Source: CAD feature listing. Evaluate the final solid. Frame: model axes, mm. A direction names the side the tool comes from. Coordinates: 2 decimals unless noted, no trailing zeros. Order: outer loops, then holes, each group sorted by start corner. A loop starts at its lowest first (then second) coordinate and runs counter-clockwise, first axis right, second up.
```python
from build123d import *

# Parameters (mm, degrees)
SKETCH1_R           = 1.25
SKETCH1_R_2         = 0.5
BOSS_EXTRUDE1_DEPTH = 6
BOSS_EXTRUDE2_DEPTH = 2
CUT_EXTRUDE1_DEPTH  = 1
CUT_EXTRUDE2_DEPTH  = 1
CUT_EXTRUDE3_DEPTH  = 2
CUT_EXTRUDE4_DEPTH  = 1
SKETCH9_R           = 1.5
CUT_EXTRUDE5_DEPTH  = 3


with BuildPart() as part:
    # Sketch1 → Boss-Extrude1 (new body)
    with BuildSketch(Plane.XY):
        with BuildLine():
            Line((2, 0), (14, 0))
            Line((14, 0), (14, 10))
            Line((14, 10), (2, 10))
            ThreePointArc((2, 10), (0.585786438, 9.414213562), (0, 8))
            Line((0, 8), (0, 2))
            ThreePointArc((0, 2), (0.585786438, 0.585786438), (2, 0))
        make_face()
        with Locations((3, 5)):
            Circle(SKETCH1_R, mode=Mode.SUBTRACT)
        with Locations((9, 8)):
            Circle(SKETCH1_R_2, mode=Mode.SUBTRACT)
        with Locations((9, 2)):
            Circle(SKETCH1_R_2, mode=Mode.SUBTRACT)
    extrude(amount=BOSS_EXTRUDE1_DEPTH)

    # Sketch2 → Boss-Extrude2 (add)
    with BuildSketch(Plane(origin=(14, 0, 0), x_dir=(0, 0, -1), z_dir=(1, 0, 0))):
        with BuildLine():
            Line((-6, 0), (-6, 10))
            Line((-6, 10), (-8, 10))
            ThreePointArc((-8, 10), (-9.414213562, 9.414213562), (-10, 8))
            Line((-10, 8), (-10, 7))
            Line((-10, 7), (-9, 7))
            ThreePointArc((-9, 7), (-7, 5), (-9, 3))
            Line((-9, 3), (-10, 3))
            Line((-10, 3), (-10, 2))
            ThreePointArc((-10, 2), (-9.414213562, 0.585786438), (-8, 0))
            Line((-8, 0), (-6, 0))
        make_face()
        with BuildLine():
            Line((-9, 7), (-10, 7))
            Line((-10, 7), (-10, 6))
            Line((-10, 6), (-9, 6))
            ThreePointArc((-9, 6), (-8, 5), (-9, 4))
            Line((-9, 4), (-10, 4))
            Line((-10, 4), (-10, 3))
            Line((-10, 3), (-9, 3))
            ThreePointArc((-9, 3), (-7, 5), (-9, 7))
        make_face()
    extrude(amount=-BOSS_EXTRUDE2_DEPTH)

    # Sketch5 → Cut-Extrude1 (cut)
    with BuildSketch(Plane.ZY.offset(-12)):
        with BuildLine():
            Line((9, 7), (11.167948086, 7))
            ThreePointArc((11.167948086, 7), (13.167948086, 5), (11.167948086, 3))
            Line((11.167948086, 3), (9, 3))
            ThreePointArc((9, 3), (7, 5), (9, 7))
        make_face()
    extrude(amount=-CUT_EXTRUDE1_DEPTH, mode=Mode.SUBTRACT)

    # Sketch6 → Cut-Extrude2 (cut)
    with BuildSketch(Plane.XY.offset(6)):
        with BuildLine():
            Line((9, 10.115579993), (9, 9.5))
            ThreePointArc((9, 9.5), (10.5, 8), (9, 6.5))
            Line((9, 6.5), (9, 3.5))
            ThreePointArc((9, 3.5), (10.5, 2), (9, 0.5))
            Line((9, 0.5), (9, -0.336498004))
            Line((9, -0.336498004), (-3.111242448, -0.336498004))
            Line((-3.111242448, -0.336498004), (-3.111242448, 10.115579993))
            Line((-3.111242448, 10.115579993), (9, 10.115579993))
        make_face()
    extrude(amount=-CUT_EXTRUDE2_DEPTH, mode=Mode.SUBTRACT)

    # Sketch7 → Cut-Extrude3 (cut)
    with BuildSketch(Plane.XY.offset(5)):
        with BuildLine():
            Line((3, 2), (-3.248762224, 2))
            ThreePointArc((-3.248762224, 2), (-6.248762224, 5), (-3.248762224, 8))
            Line((-3.248762224, 8), (3, 8))
            ThreePointArc((3, 8), (6, 5), (3, 2))
        make_face()
    extrude(amount=-CUT_EXTRUDE3_DEPTH, mode=Mode.SUBTRACT)

    # Sketch8 → Cut-Extrude4 (cut)
    with BuildSketch(Plane.XY.offset(3)):
        with BuildLine():
            Line((3, 3.75), (-1.562441064, 3.75))
            ThreePointArc((-1.562441064, 3.75), (-2.812441064, 5), (-1.562441064, 6.25))
            Line((-1.562441064, 6.25), (3, 6.25))
            ThreePointArc((3, 6.25), (4.25, 5), (3, 3.75))
        make_face()
    extrude(amount=-CUT_EXTRUDE4_DEPTH, mode=Mode.SUBTRACT)

    # Sketch9 → Cut-Extrude5 (cut)
    with BuildSketch(Plane.XY.offset(5)):
        with Locations((9, 8)):
            Circle(SKETCH9_R)
        with Locations((9, 2)):
            Circle(SKETCH9_R)
    extrude(amount=-CUT_EXTRUDE5_DEPTH, mode=Mode.SUBTRACT)


solid = part.part
```
Q1. Pull-direction query (Y, two-part tool) for faces 5 (the flat face through (8, 0, 3)), 6 (the flat face through (12.5, 7, 9.5)), 7 (the flat face through (9, 5, 5.5)); classes: pulls with the +Y half, pulls with the -Y half, needs draft (parallel to the pull), parting line crosses it, or undercut.
Solutions:
face 5: pulls with the -Y half
face 6: undercut
face 7: needs draft
Q2. Pin query (flat end, axial travel): P1, Ø1.1, axis at y = 5, z = 5.5, coming from the -X side; P2, Ø3.5, axis at x = 9, y = 8, coming from the +Z side; P3, Ø4.5, axis at y = 7, z = 9, coming from the -X side; P4, Ø1.5, axis at x = 3, y = 5, coming from the +Z side. Return the tip coordinate at first contact, or that it passes through.
Solutions:
P1: stops at x = 5.99
P2: stops at z = 6
P3: stops at x = 12
P4: passes through
Q3. Section query A-A on z = 1.25. Output: boundary loops of the cut face in (x, y), plus the area to 3 significant figures.
Solutions:
outline: (0, 2) arc R2 ccw to (2, 0) - (14, 0) - (14, 10) - (2, 10) arc R2 ccw to (0, 8) - close; hole circle Ø2.5 at (3, 5); hole circle Ø1 at (9, 2); hole circle Ø1 at (9, 8)
area: 132 mm2
Q4. Set-up query: faces 1 (the flat face through (13.2, 2.8, 10)), 2 (the flat face through (13.5, 6, 9.5)), 3 (the flat face through (11, 5, 6)), 4 (the flat face through (13, 5.03, 7.85)). Return all of +Z, -Z, +X, -X, +Y, -Y with unobstructed straight access to the full face (end or side cutting, diameter ignored); none if empty.
Solutions:
face 1: +Z, +X, -X, +Y, -Y
face 2: +Z, +X, -X
face 3: +Z, -X, +Y, -Y
face 4: +Z, -X
Q5. Material intervals for line 1 along Y through (x, z) = (9, 2.95); line 2 along Y through (x, z) = (9, 1.15); line 3 along X through (y, z) = (5, 1.6), sorted ascending.
Solutions:
line 1: y = 0 to 0.5, 3.5 to 6.5, 9.5 to 10
line 2: y = 0 to 1.5, 2.5 to 7.5, 8.5 to 10
line 3: x = 0 to 1.75, 4.25 to 14
Q6. Section query B-B on y = 5. Output: boundary loops of the cut face in (x, z), plus the area to 4 significant figures.
Solutions:
outline: (0, 0) - (1.75, 0) - (1.75, 2) - (0, 2) - close; (4.25, 0) - (14, 0) - (14, 8) - (13, 8) - (13, 7) - (12, 7) - (12, 6) - (9, 6) - (9, 5) - (6, 5) - (6, 3) - (4.25, 3) - close
area: 56.75 mm2
Q7. Section query D-D on y = 3.25. Output: boundary loops of the cut face in (x, z).
Solutions:
outline: (0, 0) - (14, 0) - (14, 10) - (13, 10) - (13, 8.03) - (12, 8.03) - (12, 6) - (9.83, 6) - (9.83, 2) - (8.17, 2) - (8.17, 5) - (5.44, 5) - (5.44, 3) - (0, 3) - close
